CAD build for the part. Positions are in the model's coordinates, mm. Face numbers are marked on the shaded views. A direction names the side the tool comes from. Give positions to 0.01 mm unless a question says otherwise; leave off trailing zeros. Write each loop counter-clockwise with the first axis right and the second up, starting at its lowest first coordinate (ties: lowest second). Pieces come first, ordered by that corner, then holes. Notation, with made-up numbers: (-24, -39.5) - (31, -39.5) arc R6 ccw to (31, -30.5) - close; hole circle Ø7 at (74, 20.25). An arc over 180 degrees is marked (long way). Answer as a JSON object with one key per item and string values.
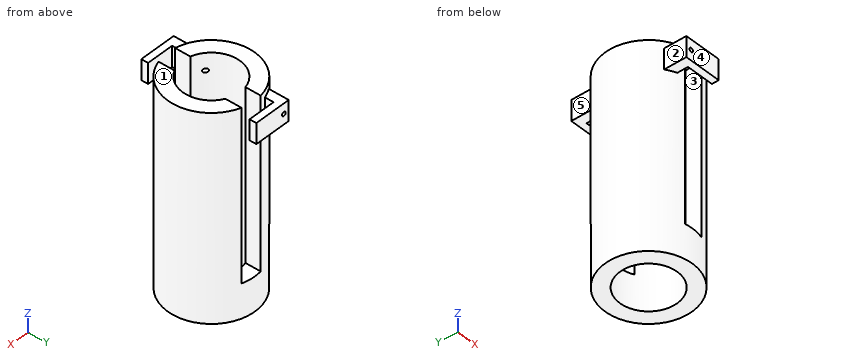
from build123d import *

# Parameters (mm, degrees)
ESBO_O1_R                     = 32
ESBO_O1_R_2                   = 21
RESSALTO_EXTRUS_O1_DEPTH      = 150
CORTE_EXTRUS_O1_DEPTH         = 167.643659607
CORTE_EXTRUS_O1_DEPTH_BACK    = 167.643659607
ESBO_O3_W                     = 125
ESBO_O3_H                     = 15
RESSALTO_EXTRUS_O2_REACH      = 168.644
RESSALTO_EXTRUS_O2_END_RADIUS = 32
ESBO_O4_W                     = 15
ESBO_O4_H                     = 7
ESBO_O5_W                     = 7
ESBO_O5_H                     = 15
RESSALTO_EXTRUS_O3_DEPTH      = 10
ESBO_O6_W                     = 15
ESBO_O6_H                     = 5
RESSALTO_EXTRUS_O4_DEPTH      = 20
RESSALTO_EXTRUS_O5_REACH      = 172.597
RESSALTO_EXTRUS_O5_END_RADIUS = 32
ESBO_O7_W                     = 15
ESBO_O7_H                     = 7
ESBO_O8_W                     = 7
ESBO_O8_H                     = 15
RESSALTO_EXTRUS_O6_DEPTH      = 10
ESBO_O9_W                     = 15
ESBO_O9_H                     = 5
RESSALTO_EXTRUS_O7_DEPTH      = 20
CORTE_EXTRUS_O2_DEPTH         = 176.206236165
CORTE_EXTRUS_O2_DEPTH_BACK    = 176.206236165
ESBO_O10_R                    = 1.5


with BuildPart() as part:
    # Esboço1 → Ressalto-extrusão1 (new body)
    with BuildSketch(Plane.XY):
        Circle(ESBO_O1_R)
        Circle(ESBO_O1_R_2, mode=Mode.SUBTRACT)
    extrude(amount=RESSALTO_EXTRUS_O1_DEPTH)

    # Esboço3 → Corte-extrusão1 (cut, two sides: drawn at the far end of the back side and taken through both)
    with BuildSketch(Plane(origin=(0, -33.162176816, 0), x_dir=(0, 0, -1), z_dir=(0, -1, 0)).offset(-CORTE_EXTRUS_O1_DEPTH_BACK)):
        with Locations((-87.5, 2.034407051)):
            Rectangle(ESBO_O3_W, ESBO_O3_H)
    extrude(amount=CORTE_EXTRUS_O1_DEPTH + CORTE_EXTRUS_O1_DEPTH_BACK, mode=Mode.SUBTRACT)

    # Ressalto-extrusão2: up to this cylinder (the profile starts outside it)
    ressalto_extrus_o2_end = Plane(origin=(0, 0, 137.5), z_dir=(0, 0, -1)) * Cylinder(RESSALTO_EXTRUS_O2_END_RADIUS, 402.288, mode=Mode.PRIVATE)
    # Esboço4 → Ressalto-extrusão2 (add, up to the surface)
    with BuildSketch(Plane(origin=(0, -33.162176816, 0), x_dir=(0, 0, -1), z_dir=(0, -1, 0)), mode=Mode.PRIVATE) as ressalto_extrus_o2_sk1:
        with Locations((-137.5, -13.965592949)):
            Rectangle(ESBO_O4_W, ESBO_O4_H)
    ressalto_extrus_o2_tool1 = extrude(ressalto_extrus_o2_sk1.sketch, amount=-RESSALTO_EXTRUS_O2_REACH, mode=Mode.PRIVATE) - ressalto_extrus_o2_end
    add(ressalto_extrus_o2_tool1.solids().sort_by_distance((-13.965593, -33.162177, 137.5))[0])

    # Esboço5 → Ressalto-extrusão3 (add)
    with BuildSketch(Plane.XZ.offset(33.162176816)):
        with Locations((-13.965592949, 137.5)):
            Rectangle(ESBO_O5_W, ESBO_O5_H)
    extrude(amount=RESSALTO_EXTRUS_O3_DEPTH)

    # Esboço6 → Ressalto-extrusão4 (add)
    with BuildSketch(Plane(origin=(-10.465592949, 0, 0), x_dir=(0, 0, -1), z_dir=(1, 0, 0))):
        with Locations((-137.5, -40.662176816)):
            Rectangle(ESBO_O6_W, ESBO_O6_H)
    extrude(amount=RESSALTO_EXTRUS_O4_DEPTH)

    # Ressalto-extrusão5: up to this cylinder (the profile starts outside it)
    ressalto_extrus_o5_end = Plane(origin=(0, 0, 137.5), z_dir=(0, 0, -1)) * Cylinder(RESSALTO_EXTRUS_O5_END_RADIUS, 410.194, mode=Mode.PRIVATE)
    # Esboço7 → Ressalto-extrusão5 (add, up to the surface)
    with BuildSketch(Plane.ZX.offset(31.532717901), mode=Mode.PRIVATE) as ressalto_extrus_o5_sk1:
        with Locations((137.5, -13.965592949)):
            Rectangle(ESBO_O7_W, ESBO_O7_H)
    ressalto_extrus_o5_tool1 = extrude(ressalto_extrus_o5_sk1.sketch, amount=-RESSALTO_EXTRUS_O5_REACH, mode=Mode.PRIVATE) - ressalto_extrus_o5_end
    add(ressalto_extrus_o5_tool1.solids().sort_by_distance((-13.965593, 31.532718, 137.5))[0])

    # Esboço8 → Ressalto-extrusão6 (add)
    with BuildSketch(Plane(origin=(0, 31.532717901, 0), x_dir=(1, 0, 0), z_dir=(0, 1, 0))):
        with Locations((-13.965592949, -137.5)):
            Rectangle(ESBO_O8_W, ESBO_O8_H)
    extrude(amount=RESSALTO_EXTRUS_O6_DEPTH)

    # Esboço9 → Ressalto-extrusão7 (add)
    with BuildSketch(Plane(origin=(-10.465592949, 0, 0), x_dir=(0, 0, -1), z_dir=(1, 0, 0))):
        with Locations((-137.5, 39.032717901)):
            Rectangle(ESBO_O9_W, ESBO_O9_H)
    extrude(amount=RESSALTO_EXTRUS_O7_DEPTH)

    # Esboço10 → Corte-extrusão2 (cut, two sides: drawn at the far end of the back side and taken through both)
    with BuildSketch(Plane.XZ.offset(43.162176816).offset(-CORTE_EXTRUS_O2_DEPTH_BACK)):
        with Locations((-13.4052452, 137.5)):
            Circle(ESBO_O10_R)
    extrude(amount=CORTE_EXTRUS_O2_DEPTH + CORTE_EXTRUS_O2_DEPTH_BACK, mode=Mode.SUBTRACT)


solid = part.part
(1) Saw through at C-C, the plane y = 0. Give the cut face in (x, z).
Answer key:
{"outline": "(-32, 0) - (-21, 0) - (-21, 150) - (-32, 150) - close; (21, 0) - (32, 0) - (32, 150) - (21, 150) - close"}
(2) Saw through at B-B, the plane z = 46. Give the cut face in (x, y), and give its area (3 significant figures).
Answer key:
{"outline": "(-5.47, -31.53) - (-5.47, -20.28) arc R21 cw to (-5.47, 20.28) - (-5.47, 31.53) arc R32 ccw to start; (9.53, -30.55) arc R32 ccw to (9.53, 30.55) - (9.53, 18.71) arc R21 cw to (9.53, -18.71) - close", "area": "1,500 mm²"}
(3) Flat gauge pins, fed straight in: P1, Ø7.5, axis at y = -33, z = 135.5, coming from the -X side; P2, Ø6, axis at y = 27, z = 89, coming from the +X side; P3, Ø8, axis at y = -25.5, z = 66, coming from the +X side; P4, Ø2.5, axis at x = -13.41, z = 137.5, coming from the +Y side. Where does each tip first touch, or does it go through?
Answer key:
{"P1": "stops at x = -17.47", "P2": "stops at x = 21.17", "P3": "stops at x = 23.7", "P4": "passes through"}
(4) Saw through at D-D, the plane z = 137.5. Give the cut face in (x, y).
Answer key:
{"outline": "(-17.47, -43.16) - (-14.91, -43.16) - (-14.91, -14.79) arc R21 cw to (-14.91, 14.79) - (-14.91, 41.53) - (-17.47, 41.53) - (-17.47, 26.81) arc R32 ccw to (-17.47, -26.81) - close; (-11.91, -43.16) - (9.53, -43.16) - (9.53, -38.16) - (-10.47, -38.16) - (-10.47, -30.24) arc R32 ccw to (-5.47, -31.53) - (-5.47, -20.28) arc R21 cw to (-11.91, -17.3) - close; (-11.91, 17.3) arc R21 cw to (-5.47, 20.28) - (-5.47, 31.53) arc R32 ccw to (-10.47, 30.24) - (-10.47, 36.53) - (9.53, 36.53) - (9.53, 41.53) - (-11.91, 41.53) - close; (9.53, -30.55) arc R32 ccw to (9.53, 30.55) - (9.53, 18.71) arc R21 cw to (9.53, -18.71) - close"}
(5) Probe L1, parallel to X at y = 29, z = 137.5; L2, parallel to X at y = 0, z = 41; L3, parallel to X at y = -35.5, z = 137.5. List the from-to ranges inside material, lowest first. Write a range as [from, to].
Answer key:
{"L1": "x = [-17.47, -14.91], [-11.91, -5.47], [9.53, 13.53]", "L2": "x = [-32, -21], [21, 32]", "L3": "x = [-17.47, -14.91], [-11.91, -10.47]"}
(6) 3-axis set-ups, long thin cutter, end or side, ignore diameter. For the marked faces 1 and 2: which of +Z, -Z, +X, -X, +Y, -Y reach the whole face in a straight line?
Answer key:
{"face 1": "+Z, +X, -X, +Y, -Y", "face 2": "+Z, -Z, -X, -Y"}
(7) Saw through at A-A, the plane x = 0. Give the cut face in (y, z), and give its area (3 significant figures).
Answer key:
{"outline": "(-43.16, 130) - (-38.16, 130) - (-38.16, 145) - (-43.16, 145) - close; (-32, 0) - (-21, 0) - (-21, 25) - (-32, 25) - close; (21, 0) - (32, 0) - (32, 25) - (21, 25) - close; (36.53, 130) - (41.53, 130) - (41.53, 145) - (36.53, 145) - close", "area": "700 mm²"}
(8) Pull direction X, two halves, no side cores. Call the marked faces 3, 4 and 5: pulls with the +X half, pulls with the -X half, needs draft (parallel to the pull), parting line crosses it, or undercut.
Answer key:
{"face 3": "undercut", "face 4": "needs draft", "face 5": "pulls with the -X half"}
